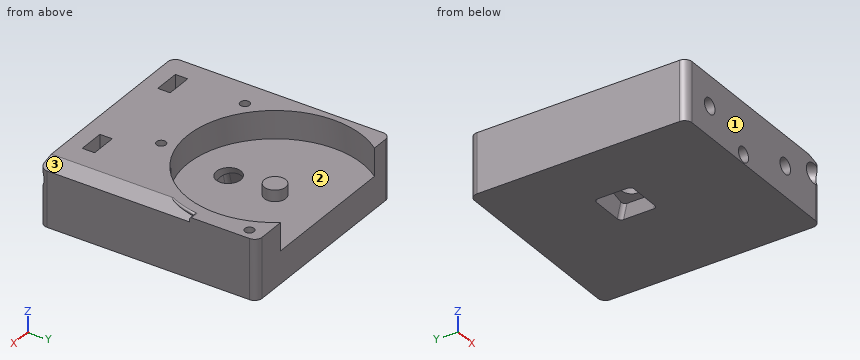
```python
from build123d import *

# Parameters (mm, degrees)
BOSS_EXTRUDE1_DEPTH      = 4
BOSS_EXTRUDE1_DEPTH_BACK = 12
SKETCH1_W                = 53
SKETCH1_H                = 58
CUT_EXTRUDE1_DEPTH       = 4
CUT_EXTRUDE1_DEPTH_BACK  = 3.4
SKETCH2_R                = 23.3
SKETCH3_R                = 2.85
BOSS_EXTRUDE2_DEPTH      = 3
SKETCH4_R                = 2.25
CUT_EXTRUDE2_DEPTH       = 32
SKETCH5_R                = 2.6
CUT_EXTRUDE3_DEPTH       = 30
SKETCH6_R                = 3.25
CUT_EXTRUDE4_DEPTH       = 44.462627624
CUT_EXTRUDE5_DEPTH       = 8
SKETCH11_R               = 1.5
CUT_EXTRUDE6_DEPTH       = 27
SKETCH12_R               = 2
CUT_EXTRUDE7_DEPTH       = 27
SKETCH13_R               = 1.25
CUT_EXTRUDE8_DEPTH       = 10
FILLET1_R                = 2
CUT_EXTRUDE9_DEPTH       = 40
BOSS_EXTRUDE3_START      = -3
BOSS_EXTRUDE3_DEPTH      = 3
FILLET3_R                = 0.5
CUT_EXTRUDE11_DEPTH      = 1.65
CUT_EXTRUDE12_REACH      = 67.513
SKETCH18_R               = 2.1


with BuildPart() as part:
    # Sketch1 → Boss-Extrude1 (new, two sides: drawn at the far end of the back side and taken through both)
    with BuildSketch(Plane.XY.offset(-BOSS_EXTRUDE1_DEPTH_BACK)):
        with Locations((1.5, -2)):
            Rectangle(SKETCH1_W, SKETCH1_H)
    extrude(amount=BOSS_EXTRUDE1_DEPTH + BOSS_EXTRUDE1_DEPTH_BACK)

    # Sketch2 → Cut-Extrude1 (cut, two sides: drawn at the far end of the back side and taken through both)
    with BuildSketch(Plane.XY.offset(-CUT_EXTRUDE1_DEPTH_BACK)):
        with Locations((0, 13)):
            Circle(SKETCH2_R)
    extrude(amount=CUT_EXTRUDE1_DEPTH + CUT_EXTRUDE1_DEPTH_BACK, mode=Mode.SUBTRACT)

    # Sketch3 → Boss-Extrude2 (add)
    with BuildSketch(Plane.XY.offset(-3.4)):
        with Locations((0, 13)):
            Circle(SKETCH3_R)
    extrude(amount=BOSS_EXTRUDE2_DEPTH)

    # Sketch4 → Cut-Extrude2 (cut)
    with BuildSketch(Plane(origin=(21.370834875, -37.015371804, 0), x_dir=(0, 0, 1), z_dir=(-0.500000000000001, 0.866025403784438, 0))):
        with Locations(Location((0, 6.5, 0), (0, 0, 90))):
            Circle(SKETCH4_R)
    extrude(amount=CUT_EXTRUDE2_DEPTH, mode=Mode.SUBTRACT)

    # Sketch5 → Cut-Extrude3 (cut)
    with BuildSketch(Plane(origin=(21.370834875, -37.015371804, 0), x_dir=(0, 0, 1), z_dir=(-0.500000000000001, 0.866025403784438, 0))):
        with Locations(Location((0, 6.5, 0), (0, 0, 120.129971207))):
            Circle(SKETCH5_R)
    extrude(amount=CUT_EXTRUDE3_DEPTH, mode=Mode.SUBTRACT)

    # Sketch6 → Cut-Extrude4 (cut, through all)
    with BuildSketch(Plane(origin=(0, 0, 0), x_dir=(0, -1, 0), z_dir=(0.25881904510252135, 0, 0.9659258262890681))):
        with Locations(Location((0, 0, 0), (0, 0, 90))):
            Circle(SKETCH6_R)
    extrude(amount=-CUT_EXTRUDE4_DEPTH, mode=Mode.SUBTRACT)

    # Sketch10 → Cut-Extrude5 (cut)
    with BuildSketch(Plane(origin=(-3.623466631, 0, -13.522961568), x_dir=(0, -1, 0), z_dir=(0.25881904510252135, 0, 0.9659258262890681))):
        with BuildLine():
            Line((4, 5), (-4, 5))
            ThreePointArc((-4, 5), (-4.707106781, 4.707106781), (-5, 4))
            Line((-5, 4), (-5, -4))
            ThreePointArc((-5, -4), (-4.707106781, -4.707106781), (-4, -5))
            Line((-4, -5), (4, -5))
            ThreePointArc((4, -5), (4.707106781, -4.707106781), (5, -4))
            Line((5, -4), (5, 4))
            ThreePointArc((5, 4), (4.707106781, 4.707106781), (4, 5))
        make_face()
    extrude(amount=CUT_EXTRUDE5_DEPTH, mode=Mode.SUBTRACT)

    # Sketch11 → Cut-Extrude6 (cut)
    with BuildSketch(Plane.XZ.offset(31)):
        with Locations(Location((-2.588190451, -9.659258263, 0), (0, 0, 270))):
            Circle(SKETCH11_R)
    extrude(amount=-CUT_EXTRUDE6_DEPTH, mode=Mode.SUBTRACT)

    # Sketch12 → Cut-Extrude7 (cut)
    with BuildSketch(Plane.XZ.offset(31)):
        with Locations(Location((-2.588190451, -9.659258263, 0), (0, 0, 270))):
            Circle(SKETCH12_R)
    extrude(amount=-CUT_EXTRUDE7_DEPTH, mode=Mode.SUBTRACT)

    # Sketch13 → Cut-Extrude8 (cut)
    with BuildSketch(Plane.XY.offset(4)):
        with Locations((25.079872408, 23)):
            Circle(SKETCH13_R)
        with Locations((-18, -7.124611797)):
            Circle(SKETCH13_R)
        with Locations((6, -13.324893162)):
            Circle(SKETCH13_R)
    extrude(amount=-CUT_EXTRUDE8_DEPTH, mode=Mode.SUBTRACT)

    # Fillet1
    # the kernel refuses this fillet: 2 mm, written as the material it takes off along each edge
    with BuildSketch(Plane(origin=(28, -31, 9), x_dir=(0, 1, 0), z_dir=(0, 0, -1))) as fillet1_piece_1:
        with BuildLine():
            CenterArc((FILLET1_R, -FILLET1_R), FILLET1_R, 90, 90)
            Line((0, -FILLET1_R), (0, 0))
            Line((0, 0), (FILLET1_R, 0))
        make_face()
    extrude(amount=12.694895612, mode=Mode.SUBTRACT)
    with BuildSketch(Plane(origin=(-25, 27, -17), x_dir=(1, 0, 0), z_dir=(0, 0, 1)), Plane(origin=(28, 27, 9), x_dir=(-1, 0, 0), z_dir=(0, 0, -1)), Plane(origin=(-25, -31, -17), x_dir=(0, 1, 0), z_dir=(0, 0, 1))) as fillet1_piece_2:
        with BuildLine():
            CenterArc((FILLET1_R, -FILLET1_R), FILLET1_R, 90, 90)
            Line((0, -FILLET1_R), (0, 0))
            Line((0, 0), (FILLET1_R, 0))
        make_face()
    extrude(amount=26, mode=Mode.SUBTRACT)
    with BuildSketch(Plane(origin=(28, -31, 3.694895612), x_dir=(0, 1, 0), z_dir=(0, 0, -1))) as fillet1_piece_3:
        with BuildLine():
            CenterArc((FILLET1_R, -FILLET1_R), FILLET1_R, 90, 90)
            Line((0, -FILLET1_R), (0, 0))
            Line((0, 0), (FILLET1_R, 0))
        make_face()
    extrude(amount=20.694895612, mode=Mode.SUBTRACT)

    # Sketch14 → Cut-Extrude9 (cut)
    with BuildSketch(Plane.XZ.offset(31)):
        Polygon((23.3, 4), (28, 2.740638796), (28, 4), align=None)
    extrude(amount=-CUT_EXTRUDE9_DEPTH, mode=Mode.SUBTRACT)

    # Sketch15 → Boss-Extrude3 (add)
    with BuildSketch(Plane.XY.offset(4).offset(BOSS_EXTRUDE3_START)):
        with BuildLine():
            Line((23.246505231, 11.422028337), (26.452977251, 11.422028337))
            ThreePointArc((26.452977251, 11.422028337), (25.46678498, 5.672458614), (23.246505231, 0.277972073))
            Line((23.246505231, 0.277972073), (20.59705621, 2.107283375))
            ThreePointArc((20.59705621, 2.107283375), (22.41105951, 6.625487343), (23.246505231, 11.422028337))
        make_face()
    extrude(amount=BOSS_EXTRUDE3_DEPTH)

    # Fillet3
    fillet3_edges = [part.edges().sort_by_distance(p)[0] for p in [
        (27.098186897, 9, 4),
        (25.121010739, 4.562890339, 4),
    ]]
    fillet(fillet3_edges, radius=FILLET3_R)

    # Sketch17 → Cut-Extrude11 (cut, symmetric)
    with BuildSketch(Plane(origin=(0, -25, 0), x_dir=(1, 0, 0), z_dir=(0, 1, 0))):
        Polygon((-12.5, 6.020725942), (-16, 8.041451884), (-19.5, 6.020725942), (-19.5, 1.979274058), (-19.5, -4), (-12.5, -4), (-12.5, 1.979274058), align=None)
        Polygon((17.5, 6.020725942), (14, 8.041451884), (10.5, 6.020725942), (10.5, 1.979274058), (10.5, -4), (17.5, -4), (17.5, 1.979274058), align=None)
    extrude(amount=CUT_EXTRUDE11_DEPTH, both=True, mode=Mode.SUBTRACT)

    # Sketch18 → Cut-Extrude12 (cut, up to next)
    with BuildSketch(Plane.XZ.offset(31), mode=Mode.PRIVATE) as cut_extrude12_sk1:
        with Locations(Location((-16, -4, 0), (0, 0, 270))):
            Circle(SKETCH18_R)
    cut_extrude12_tool1 = extrude(cut_extrude12_sk1.sketch, amount=-CUT_EXTRUDE12_REACH, mode=Mode.PRIVATE) & part.part
    # Sketch18 → Cut-Extrude12 (cut, up to next)
    with BuildSketch(Plane.XZ.offset(31), mode=Mode.PRIVATE) as cut_extrude12_sk2:
        with Locations(Location((14, -4, 0), (0, 0, 270))):
            Circle(SKETCH18_R)
    cut_extrude12_tool2 = extrude(cut_extrude12_sk2.sketch, amount=-CUT_EXTRUDE12_REACH, mode=Mode.PRIVATE) & part.part
    add(cut_extrude12_tool1.solids().sort_by_distance((-16, -31, -4))[0], mode=Mode.SUBTRACT)
    add(cut_extrude12_tool2.solids().sort_by_distance((14, -31, -4))[0], mode=Mode.SUBTRACT)


solid = part.part
```
Work out the finished part from the listing and answer in its coordinate system (mm). Face numbers are marked on the shaded views. A direction names the side the tool comes from. Give positions to 0.01 mm unless a question says otherwise; leave off trailing zeros. Order: outer loops, then holes, each group sorted by start corner. A loop starts at its lowest first (then second) coordinate and runs counter-clockwise, first axis right, second up. Notation, with made-up numbers: (23.5, 24.5) - (79.5, 24.5) arc R14 ccw to (79.5, 41.5) - close; hole circle Ø3 at (49.25, -30). An arc over 180 degrees is marked (long way). One line per item, written item: value. Start each with the question number.
1. Section C-C, the plane y = -16 is taken. Count the separate pieces of the cut face and the enclosed holes in it, then the cut area to 3 significant figures.
2. Which of the six approach directions +Z, -Z, +X, -X, +Y, -Y give full straight-line access (tool end or side, diameter ignored) to the marked faces 1, 2 and 3?
3. Section D-D, the plane y = 21 is taken. Write down the section's boundary in (x, z).
4. Each of these flat-tipped pins is pushed along its axis until it touches: pin 1 Ø3 at (x, y) = (0, 14) entering from +Z; pin 2 Ø2 at (x, y) = (-18, -7.12) entering from +Z; pin 3 Ø8 at (x, z) = (-2, -8.5) entering from -Y. Where does it stop, or does it pass through?
5. Consider line 1 (X direction, y = -28, z = -4); line 2 (Y direction, x = -18, z = -4.75); line 3 (Y direction, x = 6, z = -3.5). Determine where each line is inside the solid, lowest interval first.
6. Section B-B, the plane x = 6 is taken. Write down the section's boundary in (y, z).
7. Section A-A, the plane y = 13 is taken. Write down the section's boundary in (x, z), then the cut area to 3 significant figures.
Filled sheet:
1. separate pieces: 1
1. enclosed holes: 2
1. area: 808 mm²
2. face 1: +Z, -Z, +X, -X, -Y
2. face 2: +Z
2. face 3: +Z, +X, -Y
3. outline: (-25, -12) - (28, -12) - (28, 4) - (21.88, 4) - (21.88, -3.4) - (-21.88, -3.4) - (-21.88, 4) - (-25, 4) - close
4. pin 1: z = -0.4
4. pin 2: z = -6
4. pin 3: y = -31
5. line 1: -25 to -18.1, -13.9 to 11.9, 16.1 to 28
5. line 2: -31 to -26.65, -23.35 to -8.37, -5.87 to 27
5. line 3: -31 to -14.57, -12.07 to 27
6. outline: (-31, -12) - (27, -12) - (27, -3.4) - (-9.51, -3.4) - (-9.51, 4) - (-12.07, 4) - (-12.07, -6) - (-14.57, -6) - (-14.57, 4) - (-31, 4) - close
7. outline: (-25, -12) - (28, -12) - (28, 4) - (23.3, 4) - (23.3, -3.4) - (2.85, -3.4) - (2.85, -0.4) - (-2.85, -0.4) - (-2.85, -3.4) - (-23.3, -3.4) - (-23.3, 4) - (-25, 4) - close
7. area: 520 mm²
